Autodesk Inventor part; units mm, degrees
ref_plane "YZ Plane" through (0, 0, 0) normal (1, 0, 0) x (0, 1, 0)
ref_plane "XZ Plane" through (0, 0, 0) normal (0, 1, 0) x (-1, 0, 0)
ref_plane "XY Plane" through (0, 0, 0) normal (0, 0, 1) x (1, 0, 0)
sketch "Sketch1" plane through (0, 0, 0) normal (0, 0, 1) x (1, 0, 0)
  line L0 (0, 0) -> (177.8, 0)
  line L1 (177.8, 0) -> (177.8, 114.3)
  line L2 (177.8, 114.3) -> (0, 114.3)
  line L3 (0, 114.3) -> (0, 0)
  dimension "d0" = 177.8
  dimension "d1" = 114.3
extrude "Extrusion1" add sketch "Sketch1" along normal blind 2
sketch "Sketch2" plane through (0, 0, 2) normal (0, 0, 1) x (1, 0, 0)
  line L0 (0, 114.3) -> (0, 0)
  line L1 (177.8, 114.3) -> (0, 114.3)
  line L2 (177.8, 0) -> (177.8, 114.3)
  point P0 (6.35, 107.95)
  point P1 (6.35, 82.55)
  point P2 (6.35, 57.15)
  point P3 (6.35, 31.75)
  point P4 (6.35, 6.35)
  point P5 (31.75, 6.35)
  point P6 (57.15, 6.35)
  point P7 (82.55, 6.35)
  point P8 (95.25, 6.35)
  point P9 (146.05, 6.35)
  point P10 (120.65, 6.35)
  point P11 (171.45, 6.35)
  point P12 (171.45, 31.75)
  point P13 (171.45, 57.15)
  point P14 (171.45, 82.55)
  point P15 (171.45, 107.95)
  point P16 (120.65, 107.95)
  point P17 (146.05, 107.95)
  point P18 (95.25, 107.95)
  point P19 (82.55, 107.95)
  point P20 (57.15, 107.95)
  point P21 (31.75, 107.95)
  dimension "d4" = 25.4
  dimension "d5" = 6.35
  dimension "d7" = 6.35
  dimension "d8" = 25.4
  dimension "d9" = 25.4
  dimension "d10" = 25.4
  dimension "d11" = 25.4
  dimension "d12" = 25.4
  dimension "d13" = 25.4
  dimension "d14" = 6.35
  dimension "d15" = 25.4
  dimension "d16" = 25.4
  dimension "d17" = 25.4
hole "Hole1" at (6.35, 107.95, 2) at (6.35, 82.55, 2) at (6.35, 57.15, 2) at (6.35, 31.75, 2) at (6.35, 6.35, 2) at (31.75, 6.35, 2) at (57.15, 6.35, 2) at (82.55, 6.35, 2) at (95.25, 6.35, 2) at (146.05, 6.35, 2) at (120.65, 6.35, 2) at (171.45, 6.35, 2) at (171.45, 31.75, 2) at (171.45, 57.15, 2) at (171.45, 82.55, 2) at (171.45, 107.95, 2) at (120.65, 107.95, 2) at (146.05, 107.95, 2) at (95.25, 107.95, 2) at (82.55, 107.95, 2) at (57.15, 107.95, 2) at (31.75, 107.95, 2) direction (0, 0, -1) diameter 4.76 end through all
sketch "Sketch3" plane through (0, 0, 2) normal (0, 0, 1) x (1, 0, 0)
  line L0 (177.8, 114.3) -> (0, 114.3)
  line L1 (88.9, 114.3) -> (88.9, 0) construction
  line L2 (0, 0) -> (177.8, 0)
  point P0 (83.35, 86.25)
  point P1 (94.45, 86.25)
  point P2 (105.55, 86.25)
  point P3 (72.25, 86.25)
  point P4 (61.15, 86.25)
  point P5 (116.65, 86.25)
  dimension "d25" = 28.05
  dimension "d26" = 5.55
  dimension "d27" = 11.1
  dimension "d28" = 11.1
  dimension "d29" = 11.1
  dimension "d37" = 11.1
  dimension "d38" = 11.1
hole "Hole2" at (83.35, 86.25, 2) at (94.45, 86.25, 2) at (105.55, 86.25, 2) at (72.25, 86.25, 2) direction (0, 0, -1) diameter 8.7 end through all
hole "Hole3" at (116.65, 86.25, 2) at (61.15, 86.25, 2) direction (0, 0, -1) diameter 4.76 end through all
sketch "Sketch5" plane through (0, 0, 2) normal (0, 0, 1) x (1, 0, 0)
  line L0 (177.8, 114.3) -> (0, 114.3)
  line L1 (88.9, 114.3) -> (88.9, 0) construction
  circle A0 centre (88.9, 30.2) radius 4.7
  line L2 (84.95, 27.6529) -> (84.95, 32.7471)
  line L3 (92.85, 27.6529) -> (92.85, 32.7471)
  line L4 (0, 0) -> (177.8, 0)
  point P0 (88.9, 0)
  dimension "d46" = 9.4
  dimension "d47" = 7.9
  dimension "d48" = 3.95
  dimension "d49" = 30.2
extrude "Extrusion2" cut sketch "Sketch5" against normal through all contours L3 A0 L2
sketch "Sketch6" plane through (0, 0, 2) normal (0, 0, 1) x (1, 0, 0)
  circle A0 centre (144.8, 86.3) radius 4
  line L0 (177.8, 114.3) -> (0, 114.3)
  line L1 (177.8, 0) -> (177.8, 114.3)
  line L2 (141.3, 84.3635) -> (141.3, 88.2365)
  line L3 (144.8, 86.3) -> (136.6683, 78.1683)
  line L4 (144.8, 86.3) -> (144.8, 114.3)
  circle A1 centre (136.6683, 78.1683) radius 1.6
  point P0 (0, 0)
  dimension "d52" = 28
  dimension "d53" = 33
  dimension "d54" = 8
  dimension "d55" = 7.5
  dimension "d58" = 135
  dimension "d59" = 11.5
  dimension "d60" = 3.2
extrude "Extrusion3" cut sketch "Sketch6" against normal through all contours A1 | A0 L4 L3 L2 | A0 L3 L4
sketch "Sketch7" plane through (0, 0, 2) normal (0, 0, 1) x (1, 0, 0)
  line L0 (177.8, 0) -> (177.8, 114.3)
  line L1 (0, 0) -> (177.8, 0)
  point P0 (125.8, 52)
  point P1 (157.8, 52)
  point P2 (157.8, 20)
  point P3 (125.8, 20)
  dimension "d61" = 20
  dimension "d62" = 32
  dimension "d63" = 32
  dimension "d64" = 20
hole "Hole4" at (125.8, 52, 2) at (157.8, 52, 2) at (157.8, 20, 2) at (125.8, 20, 2) direction (0, 0, -1) diameter 2.459 end through all
sketch "Sketch8" plane through (0, 0, 2) normal (0, 0, 1) x (1, 0, 0)
  line L0 (177.8, 114.3) -> (0, 114.3)
  line L1 (0, 114.3) -> (0, 0)
  point P0 (20, 94.3)
  point P1 (52, 94.3)
  point P2 (52, 62.3)
  point P3 (20, 62.3)
  dimension "d72" = 32
  dimension "d73" = 32
  dimension "d74" = 20
  dimension "d75" = 20
hole "Hole5" at (20, 94.3, 2) at (52, 94.3, 2) at (52, 62.3, 2) at (20, 62.3, 2) direction (0, 0, -1) diameter 2.459 end through all
sketch "Sketch9" plane through (0, 0, 2) normal (0, 0, 1) x (1, 0, 0)
  line L0 (0, 114.3) -> (0, 0)
  line L1 (177.8, 114.3) -> (0, 114.3)
  point P0 (77, 62.3)
  dimension "d83" = 77
  dimension "d84" = 52
hole "Hole6" at (77, 62.3, 2) direction (0, 0, -1) diameter 4.76 end through all
sketch "Sketch10" plane through (0, 0, 2) normal (0, 0, 1) x (1, 0, 0)
  circle A0 centre (20, 94.3) radius 1.2295
  circle A1 centre (52, 94.3) radius 1.2295
  circle A2 centre (52, 62.3) radius 1.2295
  line L0 (20, 94.3) -> (52, 62.3)
  circle A3 centre (20, 62.3) radius 1.2295
  line L1 (20, 62.3) -> (52, 94.3)
  circle A4 centre (36, 78.3) radius 19
  line L2 (20, 62.3) -> (20, 94.3)
  line L3 (20, 94.3) -> (52, 94.3)
  line L4 (52, 94.3) -> (52, 62.3)
  line L5 (20, 62.3) -> (52, 62.3)
  circle A5 centre (125.8, 52) radius 1.2295
  circle A6 centre (157.8, 20) radius 1.2295
  line L6 (125.8, 52) -> (157.8, 20)
  line L7 (157.8, 20) -> (157.8, 52)
  line L8 (157.8, 52) -> (125.8, 52)
  circle A7 centre (125.8, 20) radius 1.2295
  line L9 (125.8, 20) -> (125.8, 52)
  line L10 (125.8, 20) -> (157.8, 52)
  line L11 (157.8, 20) -> (125.8, 20)
  circle A8 centre (141.8, 36) radius 19
  point P0 (0, 0)
  point P1 (125.8, 46.247)
  point P2 (125.8, 25.753)
  point P3 (131.553, 20)
  point P4 (152.047, 20)
  point P5 (157.8, 25.753)
  point P6 (157.8, 46.247)
  point P7 (152.047, 52)
  point P8 (131.553, 52)
  point P9 (20, 88.547)
  point P10 (20, 68.053)
  point P11 (25.753, 62.3)
  point P12 (46.247, 62.3)
  point P13 (52, 68.053)
  point P14 (52, 88.547)
  point P15 (46.247, 94.3)
  point P16 (25.753, 94.3)
  dimension "d92" = 38
  dimension "d93" = 38
extrude "Extrusion4" cut sketch "Sketch10" against normal blind 10 contours L3 A4 L1 L0 | A4 L0 L1 L2 | L1 A4 L4 L0 | L0 A4 L5 L1 | L8 A8 L10 L6 | A8 L6 L10 L9 | L10 A8 L7 L6 | L6 A8 L11 L10
properties part number "NRDZ_Fan_plate"
Design review of the part built by this model. Coordinates are the model's own, in mm. Coordinates: 2 decimals unless noted, no trailing zeros. Loops run counter-clockwise (first coordinate to the right, second up) from the corner with the lowest first, then second, coordinate; pieces in that order, holes last. Notation, with made-up numbers: (67.5, 89) -> (114.5, 89) arc R5 cw to (114.5, 96) -> close; hole circle Ø6 at (45, 46.5). An arc over 180 degrees is marked (long way). Use a Markdown table: item, result. Add a question column.
Item 1: We need section C-C, the plane z = 1.7. Count the separate pieces of the cut face and the enclosed holes in it, and give its area (3 significant figures).
Item 2: The part is to be moulded in two halves that separate along Y. For faces 1 (the flat face through (88, 58, 2)), 2 (the cylindrical face through (6.245, 84.928, 0.986)), 3 (the cylindrical face through (76.11, 84.24, 0.99)), say which applies: +Y half, -Y half, draft (parallel to the pull), parting line (faces both ways), or undercut.
Item 3: Wall thickness on L1, parallel to X at y = 57.15, z = 0.9; L2, parallel to Y at x = 6.35, z = 0.6; L3, parallel to Y at x = 57.15, z = 1.05: over which ranges is each line inside the solid? List them lowest first. Write a range as from..to.
Item 4: We need section A-A, the plane y = 73.5. Write out the cut boundary in (x, z).
Item 5: We need section B-B, the plane x = 105.55. Write out the cut boundary in (y, z).
Numbers:
| question | item | result |
|---|---|---|
| 1 | separate pieces | 1 |
| 1 | enclosed holes | 42 |
| 1 | area | 17,500 mm^2 |
| 2 | face 1 | draft |
| 2 | face 2 | undercut |
| 2 | face 3 | undercut |
| 3 | L1 | x = 0..3.97, 8.73..169.07, 173.83..177.8 |
| 3 | L2 | y = 0..3.97, 8.73..29.37, 34.13..54.77, 59.53..80.17, 84.93..105.57, 110.33..114.3 |
| 3 | L3 | y = 0..3.97, 8.73..105.57, 110.33..114.3 |
| 4 | outline | (0, 0) -> (20, 0) -> (20, 2) -> (0, 2) -> close; (52, 0) -> (177.8, 0) -> (177.8, 2) -> (52, 2) -> close |
| 5 | outline | (0, 0) -> (81.9, 0) -> (81.9, 2) -> (0, 2) -> close; (90.6, 0) -> (114.3, 0) -> (114.3, 2) -> (90.6, 2) -> close |
